from build123d import *

# Parameters (mm, degrees)
SKETCH3_R               = 15.875
SKETCH3_R_2             = 12.7
BOSS_EXTRUDE1_DEPTH     = 457.2
SKETCH4_R               = 24.687530181
CUT_EXTRUDE1_DEPTH      = 533.4
CUT_EXTRUDE2_DEPTH      = 458.750883396
CUT_EXTRUDE2_DEPTH_BACK = 458.750883396
SKETCH5_R               = 3.96875


with BuildPart() as part:
    # Sketch3 → Boss-Extrude1 (new, symmetric)
    with BuildSketch(Plane.XY):
        Circle(SKETCH3_R)
        Circle(SKETCH3_R_2, mode=Mode.SUBTRACT)
    extrude(amount=BOSS_EXTRUDE1_DEPTH, both=True)

    # Sketch4 → Cut-Extrude1 (cut)
    with BuildSketch(Plane.XY.offset(457.2)):
        Circle(SKETCH4_R)
    extrude(amount=-CUT_EXTRUDE1_DEPTH, mode=Mode.SUBTRACT)

    # Sketch5 → Cut-Extrude2 (cut, two sides: drawn at the far end of the back side and taken through both)
    with BuildSketch(Plane(origin=(0, 0, 0), x_dir=(1, 0, 0), z_dir=(0, 1, 0)).offset(-CUT_EXTRUDE2_DEPTH_BACK)):
        with Locations(Location((0, 85.725, 0), (0, 0, 270))):
            Circle(SKETCH5_R)
        with Locations(Location((0, 434.975, 0), (0, 0, 270))):
            Circle(SKETCH5_R)
    extrude(amount=CUT_EXTRUDE2_DEPTH + CUT_EXTRUDE2_DEPTH_BACK, mode=Mode.SUBTRACT)


solid = part.part
Source: CAD feature listing. Evaluate the final solid. Frame: model axes, mm. Round coordinates to 2 decimals unless told otherwise and drop trailing zeros. Loops run counter-clockwise (first coordinate to the right, second up) from the corner with the lowest first, then second, coordinate; pieces in that order, holes last.
Q1. Section B-B, the plane y = 0. Return loops of the section in (x, z) (3 decimals), plus the area to 3 significant figures.
Q2. Section C-C, the plane z = -267.5. Return loops of the section in (x, y) (3 decimals).
Q3. First-contact query: P1, Ø3, axis at x = 2.5, y = 9, coming from the -Z side; P2, Ø6, axis at y = 4.5, z = -161.5, coming from the +X side; P3, Ø12, axis at y = -8, z = -292, coming from the +X side; P4, Ø3, axis at x = 6.5, z = -297, coming from the +Y side. Flat tips, straight axial feed; report the tip coordinate or a pass-through.
Q4. Section A-A, the plane x = 0. Return loops of the section in (y, z) (3 decimals).
Q5. Ray query, line 1 (Z direction, x = 0, y = -13); line 2 (Y direction, x = 1, z = -222.5); line 3 (X direction, y = 8.5, z = -361.5). Return the intervals inside material, ascending.
Q6. Mould query, pull axis Z, two halves, no side actions, for faces 1 (the face through (1.19, -14, -81.94)), 2 (the face through (-7, 11, -76.2)), 3 (the face through (-7, 11, -457.2)). Classes: pulls with the +Z half, pulls with the -Z half, needs draft (parallel to the pull), parting line crosses it, or undercut.
Solutions:
1. outline: (-15.875, -457.2) - (-12.7, -457.2) - (-12.7, -76.2) - (-15.875, -76.2) - close; (12.7, -457.2) - (15.875, -457.2) - (15.875, -76.2) - (12.7, -76.2) - close
1. area: 2,420 mm2
2. outline: circle Ø31.75 at (0, 0); hole circle Ø25.4 at (0, 0)
3. P1: passes through
3. P2: stops at x = 15.8
3. P3: stops at x = 15.75
3. P4: stops at y = 15.07
4. outline: (-15.875, -457.2) - (-12.7, -457.2) - (-12.7, -438.944) - (-15.875, -438.944) - close; (-15.875, -431.006) - (-12.7, -431.006) - (-12.7, -89.694) - (-15.875, -89.694) - close; (-15.875, -81.756) - (-12.7, -81.756) - (-12.7, -76.2) - (-15.875, -76.2) - close; (12.7, -457.2) - (15.875, -457.2) - (15.875, -438.944) - (12.7, -438.944) - close; (12.7, -431.006) - (15.875, -431.006) - (15.875, -89.694) - (12.7, -89.694) - close; (12.7, -81.756) - (15.875, -81.756) - (15.875, -76.2) - (12.7, -76.2) - close
5. line 1: z = -457.2 to -438.94, -431.01 to -89.69, -81.76 to -76.2
5. line 2: y = -15.84 to -12.66, 12.66 to 15.84
5. line 3: x = -13.41 to -9.44, 9.44 to 13.41
6. face 1: undercut
6. face 2: pulls with the +Z half
6. face 3: pulls with the -Z half
